The listing builds one solid part. Answer for the finished solid, in the listing's coordinates (mm). Face numbers are marked on the shaded views. A direction names the side the tool comes from. Round coordinates to 2 decimals unless told otherwise and drop trailing zeros. Order: outer loops, then holes, each group sorted by start corner. A loop starts at its lowest first (then second) coordinate and runs counter-clockwise, first axis right, second up. Notation, with made-up numbers: (-34, 26) -> (4, 26) arc R32 ccw to (4, 57) -> close; hole circle Ø5 at (12.5, 39.25). An arc over 180 degrees is marked (long way). Answer in a Markdown table with one row per item. Add a question column.
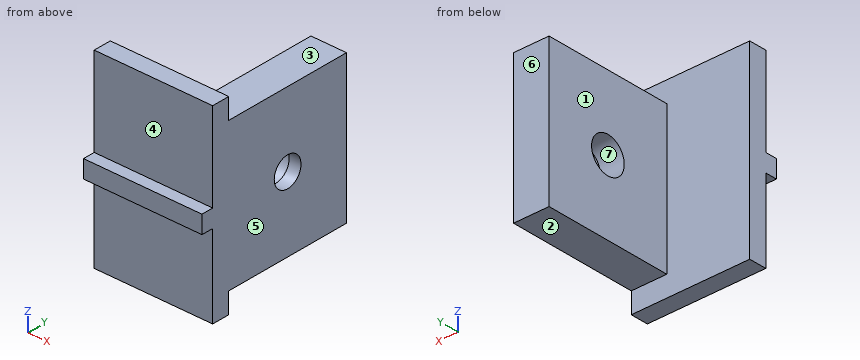
Autodesk Inventor part; units mm, degrees
ref_plane "YZ Plane" through (0, 0, 0) normal (1, 0, 0) x (0, 1, 0)
ref_plane "XZ Plane" through (0, 0, 0) normal (0, 1, 0) x (-1, 0, 0)
ref_plane "XY Plane" through (0, 0, 0) normal (0, 0, 1) x (1, 0, 0)
sketch "Sketch1" plane through (0, 0, 0) normal (1, 0, 0) x (0, 1, 0)
  line L0 (0, 0) -> (22, 0)
  line L1 (22, 0) -> (22, -25)
  line L2 (22, -25) -> (0, -25)
  line L3 (0, -25) -> (0, 0)
  circle A0 centre (11, -12.5) radius 3.05
  dimension "d0" = 22
  dimension "d1" = 25
  dimension "d2" = 6.1
  dimension "d3" = 11
  dimension "d4" = 12.5
extrude "Extrusion1" add sketch "Sketch1" along normal blind 4
sketch "Sketch2" plane through (4, 0, 0) normal (1, 0, 0) x (0, 0, -1)
  line L0 (-3.5, 0) -> (28.5, 0)
  line L1 (28.5, 0) -> (28.5, -3)
  line L2 (-3.5, -3) -> (-3.5, 0)
  line L3 (0, 22) -> (0, 0)
  line L4 (25, 0) -> (25, 22)
  line L5 (0, 0) -> (25, 0)
  line L6 (11.5, -3) -> (14.5, -3)
  line L7 (14.5, -3) -> (14.5, -5)
  line L8 (14.5, -5) -> (11.5, -5)
  line L9 (11.5, -5) -> (11.5, -3)
  line L10 (28.5, -3) -> (14.5, -3)
  line L11 (11.5, -3) -> (-3.5, -3)
  dimension "d8" = 3
  dimension "d9" = 3.5
  dimension "d10" = 3.5
  dimension "d13" = 3
  dimension "d14" = 2
  dimension "d15" = 11.5
extrude "Extrusion2" add sketch "Sketch2" along normal blind 2 and the other way blind 18
sketch "Sketch3" plane through (4, 0, 0) normal (1, 0, 0) x (0, 0, -1)
  line L0 (25, 22) -> (0, 22)
  line L1 (0, 22) -> (0, 0)
  line L2 (25, 22) -> (0, 22)
  line L3 (0, 22) -> (0, 0)
  line L4 (0, 0) -> (25, 0)
  line L5 (25, 0) -> (25, 22)
  circle A0 centre (12.5, 11) radius 2.5
  dimension "d16" = 5
  dimension "d17" = 12.5
  dimension "d18" = 11
extrude "Extrusion3" add sketch "Sketch3" along normal blind 2
equation "\"d3\" = 0.5 * d0"
properties part number "_3DPrint"
Item 1: The part is cut by section D-D, the plane z = -3. Give the vertices of the cut face in (x, y).
Item 2: Find the intervals of material crossed by probe 1 along Z at (x, y) = (2.3, 11); probe 2 along Y at (x, z) = (4.75, -12.5); probe 3 along Z at (x, y) = (1, 0.25), in increasing order. Write a range as [from, to].
Item 3: For a pull along Y with two mould halves and no side action, classify the marked faces 5, 6 and 7 as released by +Y, released by -Y, zero draft, split by the parting line, or undercut.
Item 4: The part is cut by section A-A, the plane y = 11. Give the vertices of the cut face in (x, z), and give its area (3 significant figures).
Item 5: A tool of negligible diameter and unlimited length cuts with its end or side. For the marked faces 1, 2, 3 and 4, from which of +Z, -Z, +X, -X, +Y, -Y can it reach the whole face along a straight path? Write none if from no direction.
Item 6: The part is cut by section C-C, the plane x = -3.5. Give the vertices of the cut face in (y, z), and give its area (3 significant figures).
Item 7: Flat-ended cylindrical pins translate along their axes: P1, Ø3, axis at x = 3.5, y = 3.5, coming from the +Z side; P2, Ø2, axis at x = -6, z = -24, coming from the +Y side; P3, Ø8, axis at x = 1.5, y = 18, coming from the -Z side. Find the tip coordinate at first contact, or state that the pin passes through.
Item 8: The part is cut by section B-B, the plane z = -12.5. Give the vertices of the cut face in (x, y).
Resolved:
| question | item | result |
|---|---|---|
| 1 | outline | (-14, -3) -> (6, -3) -> (6, 22) -> (0, 22) -> (0, 0) -> (-14, 0) -> close |
| 2 | probe 1 | [-25, -15.55], [-9.45, 0] |
| 2 | probe 2 | [-5, 8.5], [13.5, 22] |
| 2 | probe 3 | [-25, 0] |
| 3 | face 5 | zero draft |
| 3 | face 6 | released by +Y |
| 3 | face 7 | undercut |
| 4 | outline | (0, -25) -> (6, -25) -> (6, -15) -> (4, -15) -> (4, -15.55) -> (0, -15.55) -> close; (0, -9.45) -> (4, -9.45) -> (4, -10) -> (6, -10) -> (6, 0) -> (0, 0) -> close |
| 4 | area | 116 mm2 |
| 5 | face 1 | +Z, -Z, -X, +Y |
| 5 | face 2 | -Z, +X, -X, +Y |
| 5 | face 3 | +Z, +X, -X, +Y |
| 5 | face 4 | +Z, +X, -X, -Y |
| 6 | outline | (-5, -14.5) -> (-3, -14.5) -> (-3, -28.5) -> (0, -28.5) -> (0, 3.5) -> (-3, 3.5) -> (-3, -11.5) -> (-5, -11.5) -> close |
| 6 | area | 102 mm2 |
| 7 | P1 | z = 0 |
| 7 | P2 | y = 0 |
| 7 | P3 | z = -25 |
| 8 | outline | (-14, -5) -> (6, -5) -> (6, 8.5) -> (4, 8.5) -> (4, 7.95) -> (0, 7.95) -> (0, 0) -> (-14, 0) -> close; (0, 14.05) -> (4, 14.05) -> (4, 13.5) -> (6, 13.5) -> (6, 22) -> (0, 22) -> close |
